CAD build for the part. Positions are in the model's coordinates, mm. Give positions to 0.01 mm unless a question says otherwise; leave off trailing zeros. Loops run counter-clockwise (first coordinate to the right, second up) from the corner with the lowest first, then second, coordinate; pieces in that order, holes last.
Item 1: Probe probe 1 along X at (y, z) = (-8, -17.5); probe 2 along Z at (x, y) = (0, -12); probe 3 along X at (y, z) = (-34.5, 12). List the from-to ranges inside material, lowest first.
Item 2: Saw through at A-A on x = 6. Give the cut face in (y, z).
Item 3: Drop flat-ended pins along their axis: P1, Ø2.5, axis at x = 21, y = -31.5, coming from the -Z side; P2, Ø6.5, axis at x = -20, y = -32, coming from the +Z side; P3, Ø3, axis at x = 20, y = -32, coming from the +Z side. Give the stop position or say it passes through.
Item 4: Saw through at B-B on z = -5. Give the cut face in (x, y).
Item 5: Saw through at C-C on y = -18. Give the cut face in (x, z), plus the area to 3 significant figures.
Item 6: Saw through at D-D on y = -30.5. Give the cut face in (x, z).
from build123d import *

# Parameters (mm, degrees)
F0_W     = 52
F0_H     = 40
F1_DEPTH = 40
F2_R     = 14
F3_DEPTH = 40.001
F4_SIZE  = 12
F6_R     = 2.5
F7_DEPTH = 12
F8_R     = 2.5
F9_DEPTH = 12


with BuildPart() as f1:
    # F0 (on Front) → F1 (new body)
    with BuildSketch(Plane.XZ):
        Rectangle(F0_W, F0_H)
    extrude(amount=F1_DEPTH)

    # F2 (on face) → F3 (cut, through all)
    with BuildSketch(Plane.XZ.offset(40)):
        Circle(F2_R)
    extrude(amount=-F3_DEPTH, mode=Mode.SUBTRACT)

    # F4
    f4_edges = [f1.edges().sort_by_distance(p)[0] for p in [
        (-26, -20, 20),
        (26, -20, 20),
    ]]
    chamfer(f4_edges, length=F4_SIZE)

    # F6 (on face) → F7 (cut)
    with BuildSketch(Plane.XZ.offset(40)):
        with Locations((-19, 0)):
            Circle(F6_R)
        with Locations((-13.435029, -13.435029)):
            Circle(F6_R)
        with Locations((13.435029, -13.435029)):
            Circle(F6_R)
        with Locations((19, 0)):
            Circle(F6_R)
        with Locations((13.435029, 13.435029)):
            Circle(F6_R)
        with Locations((-13.435029, 13.435029)):
            Circle(F6_R)
    extrude(amount=-F7_DEPTH, mode=Mode.SUBTRACT)

    # F8 (on face) → F9 (cut)
    with BuildSketch(Plane(origin=(0, 0, -20), x_dir=(1, 0, 0), z_dir=(0, 0, -1))):
        with Locations((-20, 32)):
            Circle(F8_R)
        with Locations((20, 32)):
            Circle(F8_R)
        with Locations((20, 8)):
            Circle(F8_R)
        with Locations((-20, 8)):
            Circle(F8_R)
    extrude(amount=-F9_DEPTH, mode=Mode.SUBTRACT)


solid = f1.part
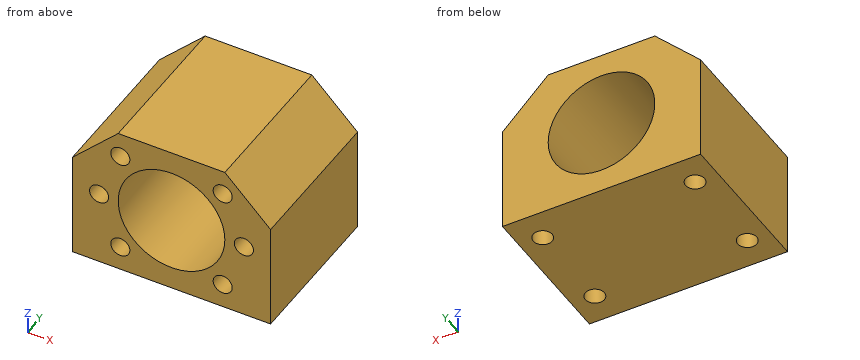
Results below:
1. probe 1: x = -26 to -22.5, -17.5 to 17.5, 22.5 to 26
1. probe 2: z = -20 to -14, 14 to 20
1. probe 3: x = -22 to -15.48, -11.39 to -7.21, 7.21 to 11.39, 15.48 to 22
2. outline: (-40, -20) - (0, -20) - (0, -12.65) - (-40, -12.65) - close; (-40, 12.65) - (0, 12.65) - (0, 20) - (-40, 20) - close
3. P1: stops at z = -8
3. P2: stops at z = 17.25
3. P3: stops at z = 15.5
4. outline: (-26, -40) - (-13.08, -40) - (-13.08, 0) - (-26, 0) - close; (13.08, -40) - (26, -40) - (26, 0) - (13.08, 0) - close
5. outline: (-26, -20) - (26, -20) - (26, 8) - (14, 20) - (-14, 20) - (-26, 8) - close; hole circle Ø28 at (0, 0)
5. area: 1,320 mm2
6. outline: (-26, -20) - (-22, -20) - (-22, -8) - (-18, -8) - (-18, -20) - (18, -20) - (18, -8) - (22, -8) - (22, -20) - (26, -20) - (26, 8) - (14, 20) - (-14, 20) - (-26, 8) - close; hole circle Ø5 at (-19, 0); hole circle Ø5 at (-13.44, -13.44); hole circle Ø5 at (-13.44, 13.44); hole circle Ø28 at (0, 0); hole circle Ø5 at (13.44, -13.44); hole circle Ø5 at (13.44, 13.44); hole circle Ø5 at (19, 0)
